Check sheet for the modelled part. Datum: model origin and axes. Units: mm. Face numbers are marked on the shaded views. Round coordinates to 2 decimals unless told otherwise and drop trailing zeros. Write each loop counter-clockwise with the first axis right and the second up, starting at its lowest first coordinate (ties: lowest second). Pieces come first, ordered by that corner, then holes. Notation, with made-up numbers: M -25.5,9.5 L 23.5,9.5 A23 ccw 23.5,42.5 Z; hole C 39.25,3 d11. An arc over 180 degrees is marked long. Answer in a Markdown table with one row per item.
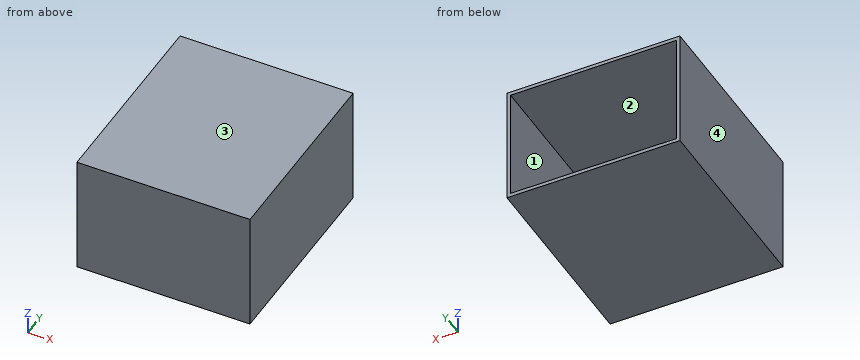
Autodesk Inventor part; units mm, degrees
ref_plane "YZ Plane" through (0, 0, 0) normal (1, 0, 0) x (0, 1, 0)
ref_plane "XZ Plane" through (0, 0, 0) normal (0, 1, 0) x (-1, 0, 0)
ref_plane "XY Plane" through (0, 0, 0) normal (0, 0, 1) x (1, 0, 0)
sketch "Boceto3" plane through (0, 0, 0) normal (0, 1, 0) x (-1, 0, 0)
  line L0 (36, -25) -> (-36, -25)
  line L1 (-36, -25) -> (-36, 25)
  line L2 (-36, 25) -> (36, 25)
  line L3 (36, 25) -> (36, -25)
  point P0 (0, 0)
  point P1 (36, 0)
  point P2 (0, -25)
  dimension "d8" = 72
  dimension "d9" = 50
extrude "Extrusión2" add sketch "Boceto3" along normal blind 82.5
sketch "Boceto5" plane through (0, 82.5, 0) normal (0, 1, 0) x (1, 0, 0)
  line L0 (-34.5, -23.5) -> (34.5, -23.5)
  line L1 (34.5, -23.5) -> (34.5, 23.5)
  line L2 (34.5, 23.5) -> (-34.5, 23.5)
  line L3 (-34.5, 23.5) -> (-34.5, -23.5)
  line L4 (-36, 25) -> (-36, -25)
  line L5 (36, 25) -> (-36, 25)
  line L6 (36, -25) -> (36, 25)
  line L7 (-36, -25) -> (36, -25)
  point P0 (0, 0)
  dimension "d12" = 1.5
  dimension "d13" = 1.5
  dimension "d14" = 1.5
  dimension "d15" = 1.5
extrude "Extrusión3" cut sketch "Boceto5" against normal blind 81 contours L3 L2 L1 L0
properties part number "Caja1_SinOrificios"
1. Go/stop test with flat-tipped pins: pin 1 (3 mm diameter, centred on x = 23, z = 10.5, fed in from +Y); pin 2 (10 mm diameter, centred on x = 4.5, z = -10.5, fed in from -Y). Record where each tip stops, or that it passes through.
Found:
| item | result |
|---|---|
| pin 1 | stops at y = 1.5 |
| pin 2 | stops at y = 0 |
2. Section check A-A, the plane y = 45.5. Record the cut outline in (x, z), and give its area (3 significant figures).
Found:
| item | result |
|---|---|
| outline | M -36,-25 L 36,-25 L 36,25 L -36,25 Z; hole M -34.5,-23.5 L 34.5,-23.5 L 34.5,23.5 L -34.5,23.5 Z |
| area | 357 mm2 |
3. Section check C-C, the plane x = 17. Record the cut outline in (y, z), and give its area (3 significant figures).
Found:
| item | result |
|---|---|
| outline | M 0,-25 L 82.5,-25 L 82.5,-23.5 L 1.5,-23.5 L 1.5,23.5 L 82.5,23.5 L 82.5,25 L 0,25 Z |
| area | 318 mm2 |
4. Draft check along Z on the marked faces 1, 2, 3 and 4. Enter one of: +Z half, -Z half, draft (parallel to the pull), parting line (faces both ways), or undercut.
Found:
| item | result |
|---|---|
| face 1 | undercut |
| face 2 | undercut |
| face 3 | +Z half |
| face 4 | draft |
5. Scan lines: L1, parallel to X at y = 30.5, z = 15.5; L2, parallel to Z at x = -5, y = 73; L3, parallel to Y at x = -6, z = -21. Record each from-to range of solid material in increasing order.
Found:
| item | result |
|---|---|
| L1 | x = -36 to -34.5, 34.5 to 36 |
| L2 | z = -25 to -23.5, 23.5 to 25 |
| L3 | y = 0 to 1.5 |
6. Section check B-B, the plane z = 6. Record the cut outline in (x, y), and give its area (3 significant figures).
Found:
| item | result |
|---|---|
| outline | M -36,0 L 36,0 L 36,82.5 L 34.5,82.5 L 34.5,1.5 L -34.5,1.5 L -34.5,82.5 L -36,82.5 Z |
| area | 351 mm2 |
